Could you check a few things on this model? Use its own coordinates, in mm. Face numbers are marked on the shaded views. A direction names the side the tool comes from. Coordinates: 2 decimals unless noted, no trailing zeros. Loops run counter-clockwise (first coordinate to the right, second up) from the corner with the lowest first, then second, coordinate; pieces in that order, holes last. Notation, with made-up numbers: (80.25, 19.5) - (112.25, 19.5) arc R31 ccw to (112.25, 54.5) - close; hole circle Ø8 at (21, -5). An arc over 180 degrees is marked (long way). Use CSV: the item, a comma, the result in double quotes.
Autodesk Inventor part; units mm, degrees
ref_plane "YZ Plane" through (0, 0, 0) normal (1, 0, 0) x (0, 1, 0)
ref_plane "XZ Plane" through (0, 0, 0) normal (0, 1, 0) x (-1, 0, 0)
ref_plane "XY Plane" through (0, 0, 0) normal (0, 0, 1) x (1, 0, 0)
sketch "Sketch1" plane through (0, 0, 0) normal (0, 1, 0) x (-1, 0, 0)
  point P0 (0, 0)
sketch "Sketch2" plane through (0, 0, 0) normal (0, 1, 0) x (-1, 0, 0)
  line L0 (-10, 34) -> (10, 34)
  line L1 (10, 34) -> (10, -34)
  line L2 (10, -34) -> (-10, -34)
  line L3 (-10, -34) -> (-10, 34)
  line L4 (-10, 34) -> (10, -34) construction
  line L5 (10, 34) -> (-10, -34) construction
  line L6 (-10, 34) -> (-25, 34)
  line L7 (-25, 34) -> (-25, -34)
  line L8 (-25, -34) -> (-10, -34)
  line L9 (-10, -34) -> (-10, 34)
  line L10 (-10, 34) -> (30, 34)
  line L11 (30, 34) -> (30, -34)
  line L12 (30, -34) -> (-10, -34)
  line L13 (-10, -34) -> (-10, 34)
  line L14 (-10, -34) -> (-14, -34)
  line L15 (-14, -34) -> (-6, -34)
  line L16 (-6, -34) -> (-14, -34)
  line L17 (-10, 34) -> (-14, 34)
  line L18 (-14, 34) -> (-6, 34)
  line L19 (-14, 34) -> (-6, 34)
  line L20 (30, 34) -> (15, 34)
  line L21 (15, 34) -> (15, -34)
  line L22 (15, -34) -> (30, -34)
  line L23 (30, -34) -> (30, 34)
  circle A0 centre (15, -34) radius 2
  circle A1 centre (15, 34) radius 2
  line L24 (15, 34) -> (19, 34)
  line L25 (19, 34) -> (11, 34)
  line L26 (11, 34) -> (11, 38)
  line L27 (11, 38) -> (19, 38)
  line L28 (19, 38) -> (19, 34)
  line L29 (15, -34) -> (19, -34)
  line L30 (19, -34) -> (11, -34)
  line L31 (11, -34) -> (11, -38)
  line L32 (11, -38) -> (19, -38)
  line L33 (19, -38) -> (19, -34)
  point P0 (0, 0)
  point P1 (10, 34)
  point P2 (13, 34)
  point P3 (17, 34)
  point P4 (17, -34)
  point P5 (13, -34)
  point P6 (10, 34)
  dimension "d0" = 20
  dimension "d1" = 68
  dimension "d4" = 15
  dimension "d5" = 40
  dimension "d10" = 4
  dimension "d11" = 8
  dimension "d42" = 15
  dimension "d43" = 4
  dimension "d44" = 4
  dimension "d45" = 4
  dimension "d46" = 8
  dimension "d47" = 4
  dimension "d48" = 8
  dimension "d49" = 4
sketch "Sketch3" plane through (0, 0, 0) normal (0, 1, 0) x (-1, 0, 0)
  point P0 (0, 0)
extrude "Extrusion1" add sketch "Sketch2" along normal blind 5 contours L0 L1 L2 L3 | L3 L8 L7 L6 | L10 A1 L21 A0 L12 L1 | L10 L21 A1 | A0 L21 L12 | L10 A1 L21 | L10 L11 L12 A0 L21 A1 | L21 A0 L12
sketch "Sketch4" plane through (0, 0, 0) normal (0, -1, 0) x (1, 0, 0)
  point P0 (0, 0)
sketch "Sketch5" plane through (-30, 0, -34) normal (-1, 0, 0) x (0, 0, 1)
  point P0 (34, 0)
sketch "Sketch6" plane through (25, 0, 34) normal (1, 0, 0) x (0, 0, -1)
  line L0 (0, -25) -> (68, -25)
  line L1 (68, -25) -> (68, 25)
  line L2 (68, 25) -> (0, 25)
  line L3 (0, 25) -> (0, -25)
  line L4 (0, -25) -> (68, 25) construction
  line L5 (68, -25) -> (0, 25) construction
  point P0 (34, 0)
  dimension "d16" = 50
  dimension "d41" = 68
extrude "Extrusion2" add sketch "Sketch6" along normal blind 5
fillet "Face Fillet1" radius 2 1 edges at (25, 5, 0)
sketch "Sketch7" plane through (30, 0, 34) normal (1, 0, 0) x (0, 0, -1)
  line L0 (68, -25) -> (68, 0)
  line L1 (0, 25) -> (68, 25)
  line L2 (68, 25) -> (68, -15)
  line L3 (68, -15) -> (0, -15)
  line L4 (0, -15) -> (0, 25)
  line L5 (0, -15) -> (32, -15)
  circle A0 centre (32, -15) radius 4
  point P0 (34, 0)
  dimension "d20" = 40
  dimension "d21" = 32
  dimension "d22" = 8
extrude "Extrusion3" cut sketch "Sketch7" against normal through all contours A0 L3 | L3 A0
sketch "Sketch8" plane through (30, 0, 34) normal (1, 0, 0) x (0, 0, -1)
  line L0 (68, -25) -> (68, 0)
  line L1 (0, 25) -> (68, 25)
  line L2 (68, 25) -> (68, -15)
  line L3 (68, -15) -> (0, -15)
  line L4 (0, -15) -> (0, 25)
  line L5 (0, -15) -> (34, -15)
  circle A0 centre (32, -15) radius 4
  line L6 (32, -15) -> (8.906, 25)
  line L7 (68, 25) -> (0, 25)
  line L8 (32, -15) -> (78.188, -15) construction
  line L9 (32, -15) -> (37.7735, -25)
  line L10 (0, -25) -> (68, -25)
  line L11 (16, 12.7128) -> (24.6603, 17.7128)
  line L12 (24.6603, 17.7128) -> (7.3397, 7.7128)
  line L13 (7.3397, 7.7128) -> (26.2265, -25)
  line L14 (26.2265, -25) -> (0, 20.4256)
  line L15 (0, 25) -> (0, -25)
  line L16 (24.6603, 17.7128) -> (49.3205, -25)
  line L17 (24.6603, 17.7128) -> (20.453, 25)
  line L18 (20.453, 25) -> (23.453, 25)
  line L19 (23.453, 25) -> (52.3205, -25)
  line L20 (26.2265, -25) -> (23.2265, -25)
  line L21 (23.2265, -25) -> (0, 15.2295)
  point P0 (34, 0)
  point P1 (0, 7)
  point P2 (0, 20.4256)
  point P3 (23.453, 25)
  point P4 (20.453, 25)
  dimension "d25" = 40
  dimension "d26" = 120
  dimension "d27" = 10
  dimension "d28" = 20
  dimension "d29" = 3
  dimension "d30" = 3
extrude "Extrusion4" add sketch "Sketch8" along normal blind 2 contours L10 L16 L3 L19 | L3 L16 L17 L1 L19 | L10 L21 L3 L13 | L3 L21 L4 L14 L13
fillet "Face Fillet2" radius 4 1 edges at (25, 0, 0)
fillet "Face Fillet3" radius 2 1 edges at (30, 0, -3.8868)
fillet "Face Fillet4" radius 2 1 edges at (30, -4.8853, 22.3868)
fillet "Fillet1" radius 2 6 edges at (-30, 2.5, -34) (-30, 2.5, 34) (27.5, -25, 34) (27.5, -25, -34) (27.5, 25, -34) (27.5, 25, 34)
extrude "Extrusion5" add sketch "Sketch2" along normal blind 5 contours L26 L27 L28 L10 A1
extrude "Extrusion6" add sketch "Sketch2" along normal blind 5 contours L12 A0 L33 L32 L31
extrude "Extrusion7" cut sketch "Sketch2" along normal blind 5 contours A0 L21 L12 | L21 A0 L12
extrude "Extrusion8" cut sketch "Sketch2" along normal blind 5 contours L10 L21 A1 | L10 A1 L21
fillet "Fillet2" radius 2 4 edges at (-19, 2.5, 38) (-11, 2.5, 38) (-19, 2.5, -38) (-11, 2.5, -38)
fillet "Face Fillet9" radius 2 1 edges at (-19, 2.5, 34)
fillet "Face Fillet10" radius 2 1 edges at (-11, 2.5, 34)
fillet "Face Fillet11" radius 2 1 edges at (-19, 2.5, -34)
fillet "Face Fillet12" radius 2 1 edges at (-11, 2.5, -34)
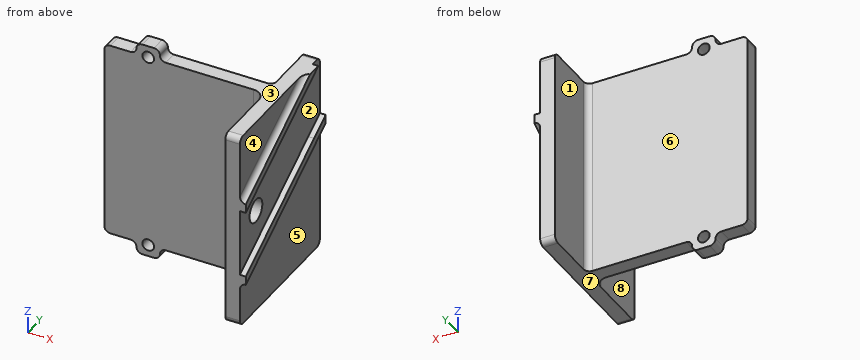
(1) Will these pins go through, and if not, where does the flat tip stop? pin 1 (12 mm diameter, centred on x = 2, y = 10.5, fed in from -Z); pin 2 (5 mm diameter, centred on x = 4, z = -17.5, fed in from +Y); pin 3 (9 mm diameter, centred on y = 16, z = 7.5, fed in from -X).
Computed:
pin 1,"stops at z = -34"
pin 2,"stops at y = 5"
pin 3,"stops at x = 25"
(2) Thinking about a two-plate mould opening in Z: for the marked faces 1, 2 and 3, which applies, +Z half, -Z half, draft (parallel to the pull), parting line (faces both ways), or undercut?
Computed:
face 1,"draft"
face 2,"undercut"
face 3,"+Z half"
(3) Which directions (+Z, -Z, +X, -X, +Y, -Y) give clear straight access to the entire face, cutting with the end or side of a thin tool? Please do the marked faces 4, 5, 6, 7 and 8.
Computed:
face 4,"+Z, +X, -Y"
face 5,"-Z, +X, +Y"
face 6,"+Z, -Z, -X, +Y"
face 7,"-Z, +X, +Y, -Y"
face 8,"+Z, -Z, -X, -Y"
(4) Please list where these lines run through material, in increasing order: line 1 (Z direction, x = -15, y = 1); line 2 (Z direction, x = 28, y = -15); line 3 (Y direction, x = 26.2, z = 2).
Computed:
line 1,"z = -38 to -36, -32 to 32, 36 to 38"
line 2,"z = -34 to -2, 6 to 34"
line 3,"y = -25 to -19, -11 to 25"
(5) Suppose I cut it at C-C (x = -18). Write out the boundary of the cut face in (y, z), plus the area to 3 significant figures.
Computed:
outline,"(0, -37.73) - (5, -37.73) - (5, 37.73) - (0, 37.73) - close"
area,"377 mm²"
(6) Suppose I cut it at A-A (z = -25). Write out the boundary of the cut face in (x, y).
Computed:
outline,"(-30, 0) - (21, 0) arc R4 cw to (25, -4) - (25, -25) - (30, -25) - (30, 25) - (25, 25) - (25, 7) arc R2 cw to (23, 5) - (-30, 5) - close"
(7) Suppose I cut it at B-B (x = -1.5). Write out the boundary of the cut face in (y, z).
Computed:
outline,"(0, -34) - (5, -34) - (5, 34) - (0, 34) - close"
